Check sheet for the modelled part. Datum: model origin and axes. Units: mm. A direction names the side the tool comes from. Coordinates: 2 decimals unless noted, no trailing zeros. Write each loop counter-clockwise with the first axis right and the second up, starting at its lowest first coordinate (ties: lowest second). Pieces come first, ordered by that corner, then holes. Notation, with made-up numbers: M 31.5,85 L 49.5,85 A27 ccw 49.5,101 Z; hole C -15,-17 d3. An arc over 180 degrees is marked long. Answer as CSV lines item,"result". Start each with the question number.
Q1. Sectioned sample at A-A, the plane x = -3.75. Record the cut outline in (y, z), then the cut area to 3 significant figures.
Q2. Sectioned sample at B-B, the plane z = 3.75. Record the cut outline in (x, y).
Q3. Sectioned sample at D-D, the plane x = -7.75. Record the cut outline in (y, z).
Q4. Thickness scan on line 1 along X through (y, z) = (9.25, 11.25); line 2 along X through (y, z) = (8.25, 3.75); line 3 along Z through (x, y) = (-11.25, 6.9). Record the ranges inside material, lowest first. Write a range as from..to.
Q5. Access from +Z, -Z, +X, -X, +Y, -Y to the whole of each face (thin tool, end or side, straight path). Record for faces 1 (the flat face through (-7.5, 9.4, 3.7)), 2 (the flat face through (-2.6, 7.05, 4.9)), 3 (the flat face through (-7.5, 13.5, 11.3)), 4 (the flat face through (-8, 4.5, 7)).
Q6. Sectioned sample at C-C, the plane y = 10.5. Record the cut outline in (x, z), then the cut area to 3 significant figures.
Q7. Mould release check, pull along Z, two halves, no side actions. Record for faces 5 (the flat face through (0, 8, 8)), 6 (the flat face through (-7, 7, 0)), 7 (the flat face through (-8, 9, 15)), 8 (the flat face through (-10, 6.05, 5)): pulls with the +Z half, pulls with the -Z half, needs draft (parallel to the pull), parting line crosses it, or undercut.
Q8. Depth check by flat-ended pin: pin 1 Ø2.5 at (x, z) = (-3.75, 11.25) entering from +Y; pin 2 Ø1.1 at (y, z) = (9.5, 2) entering from -X; pin 3 Ø4 at (x, z) = (-2.5, 10.5) entering from +Y; pin 4 Ø2.5 at (x, y) = (-9, 12) entering from -Z. Enter the tip coordinate at first touch or a pass-through.
Autodesk Inventor part; units mm, degrees
ref_plane "YZ Plane" through (0, 0, 0) normal (1, 0, 0) x (0, 1, 0)
ref_plane "XY Plane" through (0, 0, 0) normal (0, 0, 1) x (1, 0, 0)
sketch "Sketch1" plane through (0, 0, 0) normal (0, 1, 0) x (-1, 0, 0)
  line L0 (15, 15) -> (0, 15)
  line L1 (0, 15) -> (0, 0)
  line L2 (0, 0) -> (15, 0)
  line L3 (15, 0) -> (15, 15)
  dimension "d0" = 15
  dimension "d1" = 15
extrude "Extrusion1" add sketch "Sketch1" along normal blind 13
sketch "Sketch2" plane through (0, 13, 0) normal (0, 1, 0) x (1, 0, 0)
  line L0 (-15, -15) -> (0, -15) construction
  line L1 (0, -15) -> (0, 0) construction
  line L2 (0, 0) -> (-15, 0) construction
  line L3 (-15, 0) -> (-15, -15) construction
  line L4 (-15, 0) -> (-15, -15) construction
  line L5 (-15, -7.5) -> (0, -7.5) construction
  line L6 (-15, -7.5) -> (0, -7.5)
  line L7 (0, -7.5) -> (0, 0)
  line L8 (0, 0) -> (-15, 0)
  line L9 (-15, 0) -> (-15, -7.5)
extrude "Extrusion2" cut sketch "Sketch2" against normal blind 4.1
sketch "Sketch3" plane through (0, 13, 0) normal (0, 1, 0) x (1, 0, 0)
  line L0 (0, -7.5) -> (-15, -7.5) construction
  line L1 (-15, -7.5) -> (-15, -15) construction
  line L2 (-15, -15) -> (0, -15) construction
  line L3 (0, -15) -> (0, -7.5) construction
  line L4 (-15, -15) -> (0, -15) construction
  line L5 (-7.5, -15) -> (-7.5, -7.5) construction
  line L6 (-15, -15) -> (-7.5, -15)
  line L7 (-7.5, -15) -> (-7.5, -7.5)
  line L8 (-7.5, -7.5) -> (-15, -7.5)
  line L9 (-15, -7.5) -> (-15, -15)
  point P0 (0, 0)
extrude "Extrusion3" add sketch "Sketch3" along normal blind 1
sketch "Sketch4" plane through (0, 8.9, 0) normal (0, 1, 0) x (1, 0, 0)
  line L0 (0, 0) -> (0, -7.5) construction
  line L1 (-15, 0) -> (0, 0) construction
  line L2 (-15, -7.5) -> (-15, 0) construction
  line L3 (0, -7.5) -> (-15, -7.5) construction
  line L4 (-7.5, -7.5) -> (-7.5, 0) construction
  line L5 (-7.5, -7.5) -> (0, -7.5)
  line L6 (0, -7.5) -> (0, 0)
  line L7 (0, 0) -> (-7.5, 0)
  line L8 (-7.5, 0) -> (-7.5, -7.5)
extrude "Extrusion4" add sketch "Sketch4" along normal blind 1
sketch "Sketch5" plane through (0, 14, 0) normal (0, 1, 0) x (1, 0, 0)
  line L0 (-15, -15) -> (-7.5, -15) construction
  line L1 (-7.5, -15) -> (-7.5, -7.5) construction
  line L2 (-7.5, -7.5) -> (-15, -7.5) construction
  line L3 (-15, -7.5) -> (-15, -15) construction
  point P0 (0, 0)
  point P1 (-11.25, -11.25)
  point P2 (-11.25, -11.25)
sketch "Sketch6" plane through (0, 13, 0) normal (0, 1, 0) x (1, 0, 0)
  line L0 (-7.5, -7.5) -> (-7.5, -15) construction
  line L1 (-7.5, -15) -> (0, -15) construction
  line L2 (0, -15) -> (0, -7.5) construction
  line L3 (0, -7.5) -> (-7.5, -7.5) construction
  point P0 (0, 0)
  point P1 (-3.75, -11.25)
sketch "Sketch7" plane through (0, 9.9, 0) normal (0, 1, 0) x (1, 0, 0)
  line L0 (0, -7.5) -> (0, 0) construction
  line L1 (0, 0) -> (-7.5, 0) construction
  line L2 (-7.5, 0) -> (-7.5, -7.5) construction
  line L3 (0, -7.5) -> (-7.5, -7.5) construction
  point P0 (-3.75, -3.75)
sketch "Sketch8" plane through (0, 8.9, 0) normal (0, 1, 0) x (1, 0, 0)
  line L0 (-7.5, -7.5) -> (-7.5, 0) construction
  line L1 (-15, 0) -> (-7.5, 0) construction
  line L2 (-15, -7.5) -> (-15, 0) construction
  line L3 (-7.5, -7.5) -> (-15, -7.5) construction
  point P0 (0, 0)
  point P1 (-11.25, -3.75)
hole "Hole1" at (-11.25, 14, 11.25) direction (0, -1, 0) diameter 2.8448 depth 10.414 counterbore diameter 5.5 counterbore depth 2.85
hole "Hole2" at (-3.75, 13, 11.25) direction (0, -1, 0) diameter 2.8448 depth 10.414 counterbore diameter 5.5 counterbore depth 2.85
hole "Hole3" at (-11.25, 8.9, 3.75) direction (0, -1, 0) diameter 2.8448 depth 10.414 counterbore diameter 5.5 counterbore depth 2.85
hole "Hole4" at (-3.75, 9.9, 3.75) direction (0, -1, 0) diameter 2.8448 depth 10.414 counterbore diameter 5.5 counterbore depth 2.85
ref_plane "Work Plane1" through (0, 4.5, 0) normal (0, 1, 0) x (-1, 0, 0)
split "Split1" plane through (0, 4.5, 0) removes the side toward (0, -1, 0)
properties part number "screwprint"
Output:
1,outline,"M 4.5,0 L 9.9,0 L 9.9,1 L 7.05,1 L 7.05,2.33 L 4.5,2.33 Z; M 4.5,5.17 L 7.05,5.17 L 7.05,6.5 L 9.9,6.5 L 9.9,7.5 L 13,7.5 L 13,8.5 L 10.15,8.5 L 10.15,9.83 L 4.5,9.83 Z; M 4.5,12.67 L 10.15,12.67 L 10.15,14 L 13,14 L 13,15 L 4.5,15 Z"
1,area,"49.6 mm^2"
2,outline,"M -15,4.5 L -12.67,4.5 L -12.67,6.05 L -14,6.05 L -14,8.9 L -15,8.9 Z; M -9.83,4.5 L -5.17,4.5 L -5.17,7.05 L -6.5,7.05 L -6.5,9.9 L -7.5,9.9 L -7.5,8.9 L -8.5,8.9 L -8.5,6.05 L -9.83,6.05 Z; M -2.33,4.5 L 0,4.5 L 0,9.9 L -1,9.9 L -1,7.05 L -2.33,7.05 Z"
3,outline,"M 4.5,0 L 8.9,0 L 8.9,7.5 L 14,7.5 L 14,15 L 4.5,15 Z"
4,line 1,"x = -15..-12.67, -9.83..-5.17, -2.33..0"
4,line 2,"x = -15..-14, -8.5..-6.5, -1..0"
4,line 3,"z = 0..1, 6.5..9.83, 12.67..15"
5,face 1,"-Z, -X, +Y"
5,face 2,"+Y"
5,face 3,"+Z, -Z, +X, +Y"
5,face 4,"+Z, -Z, +X, -X, -Y"
6,outline,"M -15,7.5 L 0,7.5 L 0,15 L -15,15 Z; hole C -11.25,11.25 d2.84; hole C -3.75,11.25 d5.5"
6,area,"82.4 mm^2"
7,face 5,"needs draft"
7,face 6,"pulls with the -Z half"
7,face 7,"pulls with the +Z half"
7,face 8,"undercut"
8,pin 1,"passes through"
8,pin 2,"stops at x = -7.5"
8,pin 3,"stops at y = 13"
8,pin 4,"stops at z = 7.5"
